The listing builds one solid part. Answer for the finished solid, in the listing's coordinates (mm). Coordinates: 2 decimals unless noted, no trailing zeros. Order: outer loops, then holes, each group sorted by start corner. A loop starts at its lowest first (then second) coordinate and runs counter-clockwise, first axis right, second up.
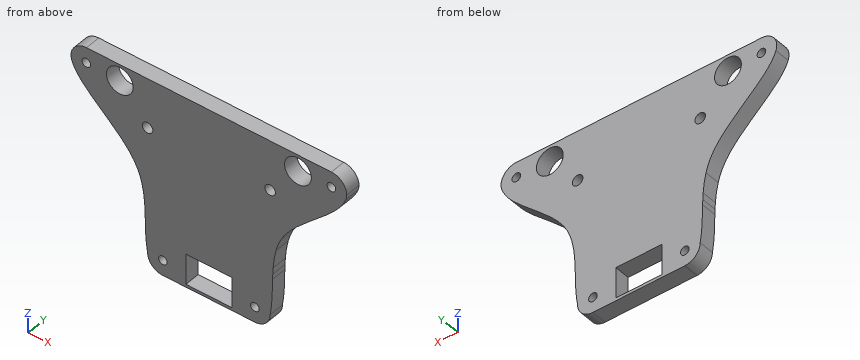
```python
from build123d import *

# Parameters (mm, degrees)
F0_R     = 7.14375
F0_R_2   = 8.73125
F0_R_3   = 22.2504
F0_W     = 76.2
F0_H     = 50.8
F1_DEPTH = 25.4


with BuildPart() as f1:
    # F0 (on Front) → F1 (new body)
    with BuildSketch(Plane.XZ):
        with BuildLine():
            ThreePointArc((-227.1798288962, 117.9559066231), (-198.9530984214, 101.2877007654), (-177.8, 126.3301412811))
            ThreePointArc((-177.8, 126.3301412811), (-185.1223559639, 144.1727528082), (-202.8676209531, 151.7279664669))
            ThreePointArc((-202.8676209531, 151.7279664669), (-223.8140359372, 141.1700038944), (-227.1798288962, 117.9559066231))
        make_face()
        with Locations((-203.2, 126.3301412811)):
            Circle(F0_R, mode=Mode.SUBTRACT)
        with BuildLine():
            ThreePointArc((-202.8676209531, 151.7279664669), (-185.1223559639, 144.1727528082), (-177.8, 126.3301412811))
            ThreePointArc((-177.8, 126.3301412811), (-198.9530984214, 101.2877007654), (-227.1798288962, 117.9559066231))
            add(Edge.make_bspline(
                [(-227.1798288962, 117.9559066231), (-213.6418582626, 78.8128585754), (-134.6303143568, 37.7909136067), (-113.6413747749, -18.1169363843), (-111.2338181852, -27.6559796071)],
                knots=[0, 0, 0, 0, 0.5134678559, 0.6154322526, 0.6154322526, 0.6154322526, 0.6154322526], degree=3))
            Line((-111.2338181852, -27.6559796071), (111.2338181852, -27.6559796071))
            add(Edge.make_bspline(
                [(227.1798288962, 117.9559066231), (213.6418582626, 78.8128585754), (134.6303143568, 37.7909136067), (113.6413747749, -18.1169363843), (111.2338181852, -27.6559796071)],
                knots=[0, 0, 0, 0, 0.5134678559, 0.6154322526, 0.6154322526, 0.6154322526, 0.6154322526], degree=3))
            ThreePointArc((227.1798288962, 117.9559066231), (182.4893469663, 111.6254192192), (203.1998639628, 151.7301412808))
            Line((203.1998639628, 151.7301412808), (-202.8676209531, 151.7279664669))
        make_face()
        with Locations((-101.6, 69.1801412811)):
            Circle(F0_R_2, mode=Mode.SUBTRACT)
        with Locations((-147.6733071194, 124.7280620759)):
            Circle(F0_R_3, mode=Mode.SUBTRACT)
        with Locations((101.6, 69.1801412811)):
            Circle(F0_R_2, mode=Mode.SUBTRACT)
        with Locations((147.6733071194, 124.7280620759)):
            Circle(F0_R_3, mode=Mode.SUBTRACT)
        with BuildLine():
            ThreePointArc((228.6, 126.3301412811), (221.1604641457, 144.2907016196), (203.1998639628, 151.7301412808))
            ThreePointArc((203.1998639628, 151.7301412808), (182.4893469663, 111.6254192192), (227.1798288962, 117.9559066231))
            ThreePointArc((227.1798288962, 117.9559066231), (228.2424405157, 122.0832397026), (228.6, 126.3301412811))
        make_face()
        with Locations((203.2, 126.3301412811)):
            Circle(F0_R, mode=Mode.SUBTRACT)
        with BuildLine():
            Line((111.2338181852, -27.6559796071), (-111.2338181852, -27.6559796071))
            add(Edge.make_bspline(
                [(-111.2338181852, -27.6559796071), (-108.6624430935, -37.8440924207), (-107.3114943085, -48.3473495809), (-106.5439984378, -59.0045117357)],
                knots=[0.6154322526, 0.6154322526, 0.6154322526, 0.6154322526, 0.7243346607, 0.7243346607, 0.7243346607, 0.7243346607], degree=3))
            ThreePointArc((-106.5439984378, -59.0045117357), (-98.7916333235, -57.5943734425), (-94.4499, -64.1698587189))
            ThreePointArc((-94.4499, -64.1698587189), (-98.4312031682, -70.5794341064), (-105.9413914893, -69.8510777735))
            add(Edge.make_bspline(
                [(-105.9413914893, -69.8510777735), (-105.8225617688, -72.7133360171), (-105.7298757075, -75.582653183), (-105.6512856578, -78.4559796071)],
                knots=[0.7611223242, 0.7611223242, 0.7611223242, 0.7611223242, 0.7901378963, 0.7901378963, 0.7901378963, 0.7901378963], degree=3))
            Line((-105.6512856578, -78.4559796071), (105.6512856578, -78.4559796071))
            add(Edge.make_bspline(
                [(105.9413914893, -69.8510777735), (105.8225617688, -72.7133360171), (105.7298757075, -75.582653183), (105.6512856578, -78.4559796071)],
                knots=[0.7611223242, 0.7611223242, 0.7611223242, 0.7611223242, 0.7901378963, 0.7901378963, 0.7901378963, 0.7901378963], degree=3))
            ThreePointArc((105.9413914893, -69.8510777735), (94.4609093557, -63.7732294435), (106.5439984378, -59.0045117357))
            add(Edge.make_bspline(
                [(111.2338181852, -27.6559796071), (108.6624430935, -37.8440924207), (107.3114943085, -48.3473495809), (106.5439984378, -59.0045117357)],
                knots=[0.6154322526, 0.6154322526, 0.6154322526, 0.6154322526, 0.7243346607, 0.7243346607, 0.7243346607, 0.7243346607], degree=3))
        make_face()
        with BuildLine():
            ThreePointArc((-94.4499, -64.1698587189), (-98.7916333235, -57.5943734425), (-106.5439984378, -59.0045117357))
            add(Edge.make_bspline(
                [(-106.5439984378, -59.0045117357), (-106.2847353017, -62.6045431988), (-106.0920508575, -66.2221369929), (-105.9413914893, -69.8510777735)],
                knots=[0.7243346607, 0.7243346607, 0.7243346607, 0.7243346607, 0.7611223242, 0.7611223242, 0.7611223242, 0.7611223242], degree=3))
            ThreePointArc((-105.9413914893, -69.8510777735), (-98.4312031682, -70.5794341064), (-94.4499, -64.1698587189))
        make_face()
        with BuildLine():
            add(Edge.make_bspline(
                [(106.5439984378, -59.0045117357), (106.2847353017, -62.6045431988), (106.0920508575, -66.2221369929), (105.9413914893, -69.8510777735)],
                knots=[0.7243346607, 0.7243346607, 0.7243346607, 0.7243346607, 0.7611223242, 0.7611223242, 0.7611223242, 0.7611223242], degree=3))
            ThreePointArc((106.5439984378, -59.0045117357), (94.4609093557, -63.7732294435), (105.9413914893, -69.8510777735))
        make_face()
        with BuildLine():
            Line((105.6512856578, -78.4559796071), (-105.6512856578, -78.4559796071))
            add(Edge.make_bspline(
                [(-105.6512856578, -78.4559796071), (-105.0828642234, -99.2380039713), (-105.2518408856, -120.2297627942), (-101.5998316324, -140.277376034)],
                knots=[0.7901378963, 0.7901378963, 0.7901378963, 0.7901378963, 1, 1, 1, 1], degree=3))
            ThreePointArc((-101.5998316324, -140.277376034), (-76.1537585809, -114.9699008108), (-50.8, -140.3698587189))
            ThreePointArc((-50.8, -140.3698587189), (-58.1440736415, -158.2344472486), (-75.9294112862, -165.7684173738))
            Line((-75.9294112862, -165.7684173738), (76.1997593484, -165.7698587177))
            ThreePointArc((76.1997593484, -165.7698587177), (58.2069048287, -122.4419886235), (101.5998316324, -140.277376034))
            add(Edge.make_bspline(
                [(105.6512856578, -78.4559796071), (105.0828642234, -99.2380039713), (105.2518408856, -120.2297627942), (101.5998316324, -140.277376034)],
                knots=[0.7901378963, 0.7901378963, 0.7901378963, 0.7901378963, 1, 1, 1, 1], degree=3))
        make_face()
        with Locations((0, -135.6059796071)):
            Rectangle(F0_W, F0_H, mode=Mode.SUBTRACT)
        with BuildLine():
            ThreePointArc((-50.8, -140.3698587189), (-76.1537585809, -114.9699008108), (-101.5998316324, -140.277376034))
            ThreePointArc((-101.5998316324, -140.277376034), (-94.2885883712, -158.2013749399), (-76.4710699897, -165.7684122419))
            Line((-76.4710699897, -165.7684122419), (-75.9294112862, -165.7684173738))
            ThreePointArc((-75.9294112862, -165.7684173738), (-58.1440736415, -158.2344472486), (-50.8, -140.3698587189))
        make_face()
        with Locations((-76.2, -140.3698587189)):
            Circle(F0_R, mode=Mode.SUBTRACT)
        with BuildLine():
            ThreePointArc((101.6, -140.3698587189), (101.5999579081, -140.3236172998), (101.5998316324, -140.277376034))
            ThreePointArc((101.5998316324, -140.277376034), (58.2069048287, -122.4419886235), (76.1997593484, -165.7698587177))
            ThreePointArc((76.1997593484, -165.7698587177), (94.1604271587, -158.330456044), (101.6, -140.3698587189))
        make_face()
        with Locations((76.2, -140.3698587189)):
            Circle(F0_R, mode=Mode.SUBTRACT)
    extrude(amount=F1_DEPTH)


solid = f1.part
```
1) A cutting plane is placed at A-A, the plane x = 15. Write down the section's boundary in (y, z).
2) A cutting plane is placed at B-B, the plane y = -9.5. Count the separate pieces of the cut face and the enclosed holes in it, plus the area to 3 significant figures.
3) Each of these flat-tipped pins is pushed along its axis until it touches: P1, Ø5, axis at y = -17, z = -5, coming from the +X side (3 decimals); P2, Ø13, axis at x = 76.2, z = -140.37, coming from the -Y side; P3, Ø2, axis at x = 148.5, y = -15.5, coming from the -Z side; P4, Ø12.5, axis at y = -7.5, z = -140.5, coming from the -X side. Where does it stop, or does it pass through?
4) Straight lines are drawn through the part: probe 1 along Z at (x, y) = (32, -14.25); probe 2 along X at (y, z) = (-15, 138); probe 3 along Z at (x, y) = (-76.2, -17.5). For each, find the intervals that lie inside material, in ascending order.
Working result:
1. outline: (-25.4, -165.77) - (0, -165.77) - (0, -161.01) - (-25.4, -161.01) - close; (-25.4, -110.21) - (0, -110.21) - (0, 151.73) - (-25.4, 151.73) - close
2. separate pieces: 1
2. enclosed holes: 9
2. area: 83,800 mm2
3. P1: stops at x = 120.805
3. P2: passes through
3. P3: stops at z = 31.78
3. P4: stops at x = -102.58
4. probe 1: z = -165.77 to -161.01, -110.21 to 151.73
4. probe 2: x = -225.76 to -165.53, -129.81 to 129.81, 165.53 to 225.76
4. probe 3: z = -165.77 to -147.51, -133.23 to 151.73
